Autodesk Inventor part; units mm, degrees
ref_plane "YZ Plane" through (0, 0, 0) normal (1, 0, 0) x (0, 1, 0)
ref_plane "XZ Plane" through (0, 0, 0) normal (0, 1, 0) x (-1, 0, 0)
ref_plane "XY Plane" through (0, 0, 0) normal (0, 0, 1) x (1, 0, 0)
sketch "Náčrt3" plane through (0, 0, 0) normal (0, 1, 0) x (-1, 0, 0)
  line L0 (-70, 45) -> (70, 45)
  line L1 (70, 45) -> (70, -45)
  line L2 (70, -45) -> (-70, -45)
  line L3 (-70, -45) -> (-70, 45)
  line L4 (-70, 45) -> (70, -45) construction
  line L5 (70, 45) -> (-70, -45) construction
  point P0 (0, 0)
  dimension "d31" = 140
  dimension "d32" = 90
extrude "Vysunutí" add sketch "Náčrt3" along normal blind 15
chamfer "Zkosení1" distance 2 angle 45 1 edges at (70, 7.5, 45)
chamfer "Zkosení2" distance 2 angle 45 1 edges at (70, 7.5, -45)
chamfer "Zkosení3" distance 2 angle 45 1 edges at (-70, 7.5, 45)
chamfer "Zkosení4" distance 2 angle 45 1 edges at (-70, 7.5, -45)
sketch "Náčrt4" plane through (0, 15, 0) normal (0, 1, 0) x (1, 0, 0)
  line L0 (68, 45) -> (-68, 45)
  line L1 (-70, 43) -> (-70, -43)
  point P0 (0, 0)
  point P1 (-55, 30)
  dimension "d47" = 15
  dimension "d48" = 15
hole "Díra" at (-55, 15, -30) direction (0, -1, 0) diameter 10 end through all counterbore diameter 20 counterbore depth 5
pattern_linear "Obdélníkové pole" count 2 spacing 110 along (1, 0, 0) count 2 spacing 60 along (0, 0, 1) of "Díra"
sketch "Náčrt5" plane through (0, 15, 0) normal (0, 1, 0) x (1, 0, 0)
  circle A0 centre (0, 0) radius 30
  dimension "d62" = 60
extrude "Vysunutí2" add sketch "Náčrt5" along normal blind 20
chamfer "Zkosení5" distance 2 angle 45 1 edges at (-30, 35, 0)
sketch "Náčrt6" plane through (0, 35, 0) normal (0, 1, 0) x (1, 0, 0)
  circle A0 centre (0, 0) radius 28
hole "Díra3" at (0, 35, 0) direction (0, -1, 0) diameter 20 end through all
sketch "Náčrt12" plane through (0, 35, 0) normal (0, 1, 0) x (1, 0, 0)
  circle A0 centre (0, 0) radius 20
  circle A1 centre (0, 20) radius 4
  dimension "d114" = 40
  dimension "d115" = 8
extrude "Vysunutí3" cut sketch "Náčrt12" against normal through all contours A1 A0 | A0 A1 picked at (0, 18.6369) picked at (0.0994, 21.2999)
pattern_circular "Kruhové pole" count 6 over 360 about axis through (0, -135.0735, 0) along (0, 1, 0) of "Vysunutí3"
properties part number "desticka"
Can you work these out from the model? Positions are in its coordinate system, mm. A direction names the side the tool comes from. Give positions to 0.01 mm unless a question says otherwise; leave off trailing zeros. Write each loop counter-clockwise with the first axis right and the second up, starting at its lowest first coordinate (ties: lowest second). Pieces come first, ordered by that corner, then holes. Notation, with made-up numbers: (74, -8.75) -> (114, -8.75) arc R19 cw to (114, 28.25) -> close; hole circle Ø10 at (24.5, 4). An arc over 180 degrees is marked (long way). Answer as a JSON object with one key per item and string values. Group by question number.
Item 1: Suppose I cut it at C-C (y = 25.5). Please give me the cut outline in (x, z), plus the area to 3 significant figures.
Item 2: I'm going to push flat-ended pins straight in: P1, Ø8, axis at y = 25, z = -31.5, coming from the +X side; P2, Ø6.5, axis at x = 17.32, z = 10, coming from the +Y side; P3, Ø1, axis at x = 54.5, z = 19.5, coming from the +Y side; P4, Ø6, axis at x = -52.5, z = -30, coming from the +Y side. Where does each tip first touch, or does it pass through?
Item 3: Suppose I cut it at B-B (x = 55). Please give me the cut outline in (y, z).
Item 4: Please list where these lines run through material, in increasing order: line 1 (X direction, y = 3, z = -30); line 2 (X direction, y = 14, z = 29.5); line 3 (Z direction, x = 55, y = 7). Write a range as [from, to].
Item 5: For faces 4 (the face through (-0.521, 17.745, -23.966)), 5 (the face through (-29.97, 23.87, 1.32)), which set-ups out of +Z, -Z, +X, -X, +Y, -Y let a thin tool reach every point of the face, with its end or its side?
Item 6: Suppose I cut it at D-D (z = 38). Please give me the cut outline in (x, y).
Item 7: Suppose I cut it at A-A (z = 0). Please give me the cut outline in (x, y).
Item 8: We'd pull the mould along Z, two halves only. Please class faces 1 (the face through (1, 7, 45)), 2 (the face through (-70, 7, 1)), 3 (the face through (-14.146, 17.745, -12.434)): +Z half, -Z half, draft (parallel to the pull), parting line (faces both ways), or undercut.
Findings:
{
 "1": {"outline": "circle Ø60 at (0, 0); hole circle Ø8 at (-17.32, -10); hole circle Ø8 at (-17.32, 10); hole circle Ø20 at (0, 0); hole circle Ø8 at (0, -20); hole circle Ø8 at (0, 20); hole circle Ø8 at (17.32, -10); hole circle Ø8 at (17.32, 10)", "area": "2,210 mm²"},
 "2": {"P1": "stops at x = 11.99", "P2": "passes through", "P3": "stops at y = 15", "P4": "stops at y = 10"},
 "3": {"outline": "(0, -45) -> (15, -45) -> (15, -40) -> (10, -40) -> (10, -35) -> (0, -35) -> close; (0, -25) -> (10, -25) -> (10, -20) -> (15, -20) -> (15, 20) -> (10, 20) -> (10, 25) -> (0, 25) -> close; (0, 35) -> (10, 35) -> (10, 40) -> (15, 40) -> (15, 45) -> (0, 45) -> close"},
 "4": {"line 1": "x = [-70, -60], [-50, 50], [60, 70]", "line 2": "x = [-70, -64.99], [-45.01, 45.01], [64.99, 70]", "line 3": "z = [-45, -35], [-25, 25], [35, 45]"},
 "5": {"face 4": "+Y, -Y", "face 5": "+Y"},
 "6": {"outline": "(-70, 0) -> (70, 0) -> (70, 15) -> (61, 15) -> (61, 10) -> (49, 10) -> (49, 15) -> (-49, 15) -> (-49, 10) -> (-61, 10) -> (-61, 15) -> (-70, 15) -> close"},
 "7": {"outline": "(-70, 0) -> (-10, 0) -> (-10, 35) -> (-28, 35) -> (-30, 33) -> (-30, 15) -> (-70, 15) -> close; (10, 0) -> (70, 0) -> (70, 15) -> (30, 15) -> (30, 33) -> (28, 35) -> (10, 35) -> close"},
 "8": {"face 1": "+Z half", "face 2": "draft", "face 3": "undercut"}
}
